Design review of the part shown in the three views and the two pictorial views. Dimensions are in mm from the part's minimum x, y and z. Round coordinates to 2 decimals unless told otherwise and drop trailing zeros. Write each loop counter-clockwise with the first axis right and the second up, starting at its lowest first coordinate (ties: lowest second). Pieces come first, ordered by that corner, then holes. Notation, with made-up numbers: (25, 89.25) -> (62, 89.25) arc R26 ccw to (62, 103.25) -> close; hole circle Ø11 at (-15, 53.25). An arc over 180 degrees is marked (long way). Answer as a JSON object with one key per item and string values. Group by question number.
1) Insertion check: pin 1 Ø2 at (x, y) = (6, 50) entering from -Z. The pin has a flat end and moves straight along its axis. Give the tip position at first contact, or say it passes through.
2) To check wall thickness, follow probe 1 along Y at (x, z) = (46, 2.8); probe 2 along Y at (x, z) = (86, 1.7); probe 3 along X at (y, z) = (48.5, 0.8). State the ranges of each line that lie inside material, in increasing order. Write a range as [from, to].
3) We need section C-C, the plane y = 28. Write out the cut boundary in (x, z), then the cut area to 3 significant figures.
4) We need section A-A, the plane x = 38. Write out the cut boundary in (y, z), then the cut area to 3 significant figures.
5) We need section B-B, the plane y = 20. Write out the cut boundary in (x, z).
6) We need section D-D, the plane z = 3.1. Count the separate pieces of the cut face and the enclosed holes in it, then the cut area to 3 significant figures.
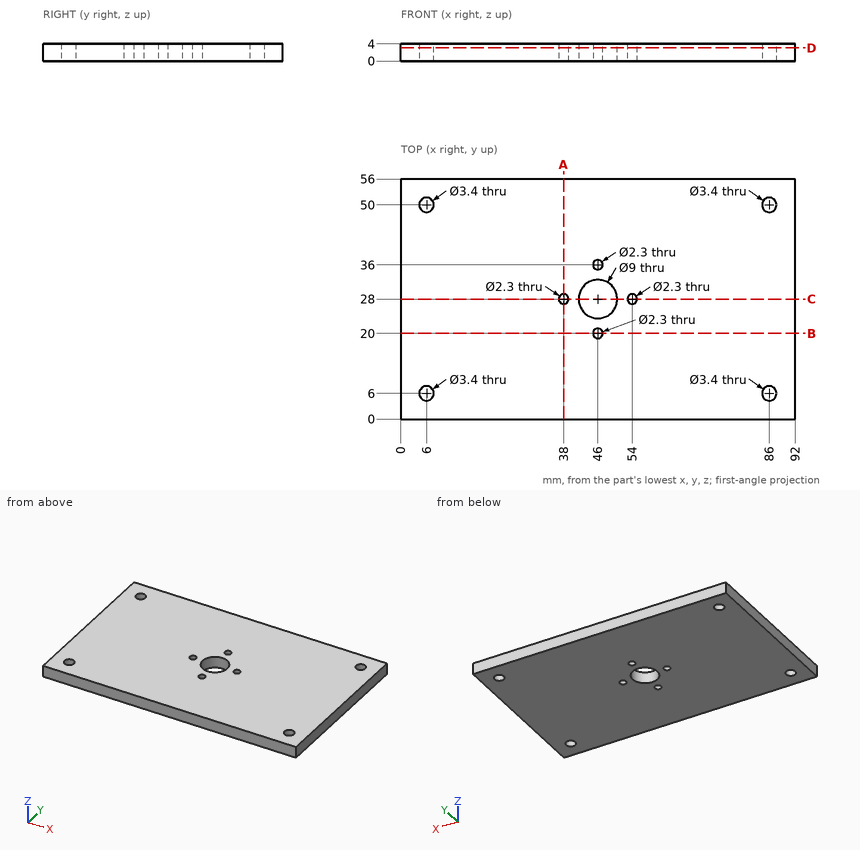
Here are the results:
{
 "1": {"pin 1": "passes through"},
 "2": {"probe 1": "y = [0, 18.85], [21.15, 23.5], [32.5, 34.85], [37.15, 56]", "probe 2": "y = [0, 4.3], [7.7, 48.3], [51.7, 56]", "probe 3": "x = [0, 5.2], [6.8, 85.2], [86.8, 92]"},
 "3": {"outline": "(0, 0) -> (36.85, 0) -> (36.85, 4) -> (0, 4) -> close; (39.15, 0) -> (41.5, 0) -> (41.5, 4) -> (39.15, 4) -> close; (50.5, 0) -> (52.85, 0) -> (52.85, 4) -> (50.5, 4) -> close; (55.15, 0) -> (92, 0) -> (92, 4) -> (55.15, 4) -> close", "area": "314 mm^2"},
 "4": {"outline": "(0, 0) -> (26.85, 0) -> (26.85, 4) -> (0, 4) -> close; (29.15, 0) -> (56, 0) -> (56, 4) -> (29.15, 4) -> close", "area": "215 mm^2"},
 "5": {"outline": "(0, 0) -> (44.85, 0) -> (44.85, 4) -> (0, 4) -> close; (47.15, 0) -> (92, 0) -> (92, 4) -> (47.15, 4) -> close"},
 "6": {"separate pieces": "1", "enclosed holes": "9", "area": "5,040 mm^2"}
}
